Input: part model. Units: mm. Frame: model coordinates. Face numbers are marked on the shaded views. Round coordinates to 2 decimals unless told otherwise and drop trailing zeros. Loops run counter-clockwise (first coordinate to the right, second up) from the corner with the lowest first, then second, coordinate; pieces in that order, holes last. Notation, with made-up numbers: (29, 69.25) - (55, 69.25) arc R16 cw to (55, 95.25) - close; hole circle Ø4 at (41, 9.5). An arc over 180 degrees is marked (long way). Use CSV: the item, a comma, the result in double quotes. Start each with the question number.
1. Cut plane A-A (y = 0). Return loops of the section in (x, z).
2. Pull-direction query (Y, two-part tool) for the marked faces 1, 2 and 3; classes: +Y half, -Y half, draft (parallel to the pull), parting line (faces both ways), or undercut.
3. Pin query (flat end, axial travel): P1, Ø3, axis at y = -13.5, z = 28.5, coming from the -X side; P2, Ø9, axis at y = 0, z = 22.86, coming from the +X side. Return the tip coordinate at first contact, or that it passes through.
4. Material intervals for probe 1 along Z at (x, y) = (83, 3.5); probe 2 along Y at (x, z) = (58, 22.86); probe 3 along Z at (x, y) = (77.5, -1.5), sorted ascending. Write a range as from..to.
5. Cut plane B-B (z = -7.62). Return loops of the section in (x, y), and give its area (3 significant figures).
6. Cut plane C-C (x = 69). Return loops of the section in (y, z), and give its area (3 significant figures).
7. Cut plane D-D (y = -10). Return loops of the section in (x, z), and give its area (3 significant figures).
```python
from build123d import *

# Parameters (mm, degrees)
SKETCH1_W           = 50.8
SKETCH1_H           = 76.2
SKETCH1_R           = 15.24
SKETCH1_R_2         = 7.62
BOSS_EXTRUDE1_DEPTH = 101.6
FILLET1_R           = 2.54
CHAMFER1_SIZE       = 2.54


with BuildPart() as part:
    # Sketch1 → Boss-Extrude1 (new body)
    with BuildSketch(Plane.YZ):
        Rectangle(SKETCH1_W, SKETCH1_H)
        with Locations(Location((0, -7.62, 0), (0, 0, 270))):
            Circle(SKETCH1_R, mode=Mode.SUBTRACT)
        with Locations(Location((0, 22.86, 0), (0, 0, 270))):
            Circle(SKETCH1_R_2, mode=Mode.SUBTRACT)
    extrude(amount=BOSS_EXTRUDE1_DEPTH)

    # Fillet1
    fillet1_edges = [part.edges().sort_by_distance(p)[0] for p in [
        (50.8, -25.4, 38.1),
        (50.8, -25.4, -38.1),
    ]]
    fillet(fillet1_edges, radius=FILLET1_R)

    # Chamfer1
    chamfer1_edges = [part.edges().sort_by_distance(p)[0] for p in [
        (50.8, 25.4, 38.1),
        (50.8, 25.4, -38.1),
    ]]
    chamfer(chamfer1_edges, length=CHAMFER1_SIZE)


solid = part.part
```
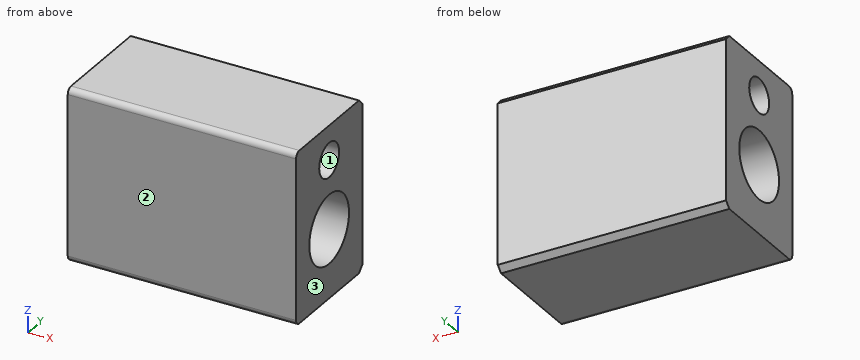
Established:
1,outline,"(0, -38.1) - (101.6, -38.1) - (101.6, -22.86) - (0, -22.86) - close; (0, 7.62) - (101.6, 7.62) - (101.6, 15.24) - (0, 15.24) - close; (0, 30.48) - (101.6, 30.48) - (101.6, 38.1) - (0, 38.1) - close"
2,face 1,"undercut"
2,face 2,"-Y half"
2,face 3,"draft"
3,P1,"stops at x = 0"
3,P2,"passes through"
4,probe 1,"z = -38.1..-22.45, 7.21..16.09, 29.63..38.1"
4,probe 2,"y = -25.4..-7.62, 7.62..25.4"
4,probe 3,"z = -38.1..-22.79, 7.55..15.39, 30.33..38.1"
5,outline,"(0, -25.4) - (101.6, -25.4) - (101.6, -15.24) - (0, -15.24) - close; (0, 15.24) - (101.6, 15.24) - (101.6, 25.4) - (0, 25.4) - close"
5,area,"2,060 mm2"
6,outline,"(-25.4, -35.56) arc R2.54 ccw to (-22.86, -38.1) - (22.86, -38.1) - (25.4, -35.56) - (25.4, 35.56) - (22.86, 38.1) - (-22.86, 38.1) arc R2.54 ccw to (-25.4, 35.56) - close; hole circle Ø30.48 at (0, -7.62); hole circle Ø15.24 at (0, 22.86)"
6,area,"2,950 mm2"
7,outline,"(0, -38.1) - (101.6, -38.1) - (101.6, -19.12) - (0, -19.12) - close; (0, 3.88) - (101.6, 3.88) - (101.6, 38.1) - (0, 38.1) - close"
7,area,"5,410 mm2"
